The model under review builds one solid part; all positions refer to its coordinate system, in mm. Face numbers are marked on the shaded views. A direction names the side the tool comes from. Round coordinates to 2 decimals unless told otherwise and drop trailing zeros. Write each loop counter-clockwise with the first axis right and the second up, starting at its lowest first coordinate (ties: lowest second). Pieces come first, ordered by that corner, then holes.
Item 1: Add section B-B (z = 0). Give the boundary of the cut face in (x, y) (3 decimals).
Item 2: Add section A-A (x = -30). Give the boundary of the cut face in (y, z) (3 decimals).
Item 3: Draft analysis for pull direction Z (two halves, no side actions). For the marked faces 3, 4 and 5, state which applies: +Z half, -Z half, draft (parallel to the pull), parting line (faces both ways), or undercut.
Item 4: Clearance check with flat-ended pins moving along their axes: pin 1 Ø1 at (x, z) = (12.5, 4) entering from -Y; pin 2 Ø5 at (x, z) = (-27.5, 2) entering from +Y. State where each tip first meets the part, or that it passes through.
Item 5: Machinability: for the marked faces 1 and 2, which of the approach directions +Z, -Z, +X, -X, +Y, -Y give a long, thin tool a straight path to every point of the face, cutting with its end or side? Answer none if there is none.
Item 6: Add section C-C (y = 5.25). Give the boundary of the cut face in (x, z) (3 decimals).
Item 7: To check wall thickness, follow L1, parallel to Z at x = -29.5, y = 3.25 (3 decimals); L2, parallel to X at y = 9.25, z = 0.5; L3, parallel to Z at x = -24.5, y = 0.5 (3 decimals). State the ranges of each line that lie inside material, in increasing order.
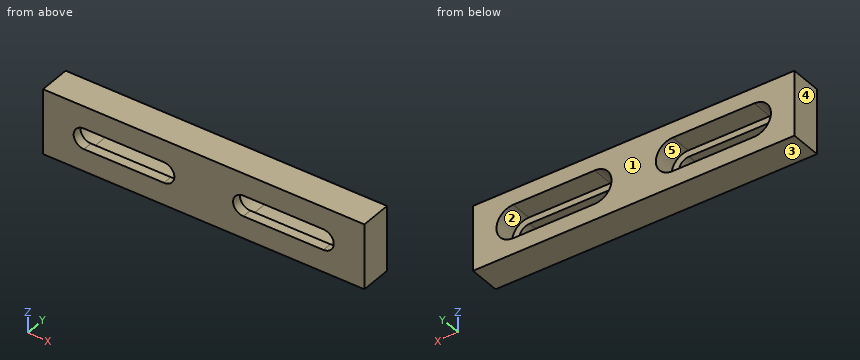
```python
from build123d import *

# Parameters (mm, degrees)
SKETCH_2_W          = 100
SKETCH_2_H          = 20.25
EXTRUDE_2_DEPTH     = 9.8
CUT_EXTRUDE_4_DEPTH = 9.8
EXTRUDE_3_DEPTH     = 3


with BuildPart() as part:
    # 草图2 → 凸台-拉伸2 (new body)
    with BuildSketch(Plane(origin=(0, 0, 0), x_dir=(1, 0, 0), z_dir=(0, 1, 0))):
        Rectangle(SKETCH_2_W, SKETCH_2_H)
    extrude(amount=EXTRUDE_2_DEPTH)

    # 草图6 → 切除-拉伸4 (cut)
    with BuildSketch(Plane(origin=(0, 0, 0), x_dir=(1, 0, 0), z_dir=(0, 1, 0))):
        with BuildLine():
            Line((-37.475, 5.225), (-12.125, 5.225))
            ThreePointArc((-12.125, 5.225), (-6.9, 0), (-12.125, -5.225))
            Line((-12.125, -5.225), (-37.475, -5.225))
            ThreePointArc((-37.475, -5.225), (-42.7, 0), (-37.475, 5.225))
        make_face()
        with BuildLine():
            Line((37.475, -5.225), (12.125, -5.225))
            ThreePointArc((12.125, -5.225), (6.9, 0), (12.125, 5.225))
            Line((12.125, 5.225), (37.475, 5.225))
            ThreePointArc((37.475, 5.225), (42.7, 0), (37.475, -5.225))
        make_face()
    extrude(amount=CUT_EXTRUDE_4_DEPTH, mode=Mode.SUBTRACT)

    # 草图8 → 凸台-拉伸3 (add)
    with BuildSketch(Plane.XZ):
        with BuildLine():
            Line((-37.475, 5.225), (-12.125, 5.225))
            ThreePointArc((-12.125, 5.225), (-6.9, 0), (-12.125, -5.225))
            Line((-12.125, -5.225), (-37.475, -5.225))
            ThreePointArc((-37.475, -5.225), (-42.7, 0), (-37.475, 5.225))
        make_face()
        with BuildLine():
            Line((-37.25, 3.215), (-12.35, 3.215))
            ThreePointArc((-12.35, 3.215), (-9.135, 0), (-12.35, -3.215))
            Line((-12.35, -3.215), (-37.25, -3.215))
            ThreePointArc((-37.25, -3.215), (-40.465, 0), (-37.25, 3.215))
        make_face(mode=Mode.SUBTRACT)
        with BuildLine():
            Line((37.475, 5.225), (12.125, 5.225))
            ThreePointArc((12.125, 5.225), (6.9, 0), (12.125, -5.225))
            Line((12.125, -5.225), (37.475, -5.225))
            ThreePointArc((37.475, -5.225), (42.7, 0), (37.475, 5.225))
        make_face()
        with BuildLine():
            Line((37.25, -3.215), (12.35, -3.215))
            ThreePointArc((12.35, -3.215), (9.135, 0), (12.35, 3.215))
            Line((12.35, 3.215), (37.25, 3.215))
            ThreePointArc((37.25, 3.215), (40.465, 0), (37.25, -3.215))
        make_face(mode=Mode.SUBTRACT)
    extrude(amount=-EXTRUDE_3_DEPTH)


solid = part.part
```
Numbers:
1. outline: (-50, 0) - (-40.465, 0) - (-40.465, 3) - (-42.7, 3) - (-42.7, 9.8) - (-50, 9.8) - close; (-9.135, 0) - (9.135, 0) - (9.135, 3) - (6.9, 3) - (6.9, 9.8) - (-6.9, 9.8) - (-6.9, 3) - (-9.135, 3) - close; (40.465, 0) - (50, 0) - (50, 9.8) - (42.7, 9.8) - (42.7, 3) - (40.465, 3) - close
2. outline: (0, -10.125) - (9.8, -10.125) - (9.8, -5.225) - (3, -5.225) - (3, -3.215) - (0, -3.215) - close; (0, 3.215) - (3, 3.215) - (3, 5.225) - (9.8, 5.225) - (9.8, 10.125) - (0, 10.125) - close
3. face 3: -Z half
3. face 4: draft
3. face 5: undercut
4. pin 1: stops at y = 0
4. pin 2: stops at y = 3
5. face 1: +Z, -Z, +X, -X, +Y
5. face 2: +Y
6. outline: (-50, -10.125) - (50, -10.125) - (50, 10.125) - (-50, 10.125) - close; hole (-37.475, -5.225) - (-12.125, -5.225) arc R5.225 ccw to (-12.125, 5.225) - (-37.475, 5.225) arc R5.225 ccw to start; hole (12.125, -5.225) - (37.475, -5.225) arc R5.225 ccw to (37.475, 5.225) - (12.125, 5.225) arc R5.225 ccw to start
7. L1: z = -10.125 to -5.225, 5.225 to 10.125
7. L2: x = -50 to -42.68, -6.92 to 6.92, 42.68 to 50
7. L3: z = -10.125 to -3.215, 3.215 to 10.125
